Work out the finished part from the listing and answer in its coordinate system (mm). A direction names the side the tool comes from. Give positions to 0.01 mm unless a question says otherwise; leave off trailing zeros. Write each question's results on one line, items separated by ' | '.
from build123d import *

# Parameters (mm, degrees)
EXTRUDE_1_DEPTH     = 5
SKETCH_2_R          = 1.5
CUT_EXTRUDE_1_DEPTH = 202.618451537


with BuildPart() as part:
    # 草圖1 → 填料-伸長1 (new body)
    with BuildSketch(Plane(origin=(0, 0, 0), x_dir=(1, 0, 0), z_dir=(0, 1, 0))):
        Polygon((173, -65), (185, -65), (185, -35), (173, -35), (173, 35), (185, 35), (185, 65), (173, 65), (173, 80), (-173, 80), (-173, 65), (-185, 65), (-185, 35), (-173, 35), (-173, -35), (-185, -35), (-185, -65), (-173, -65), (-173, -80), (173, -80), align=None)
    extrude(amount=EXTRUDE_1_DEPTH)

    # 草圖2 → 除料-伸長1 (cut, through all)
    with BuildSketch(Plane(origin=(0, 5, 0), x_dir=(1, 0, 0), z_dir=(0, 1, 0))):
        with Locations(Location((-53.75, 16.75, 0), (0, 0, 270))):
            Circle(SKETCH_2_R)
        with Locations(Location((53.75, 16.75, 0), (0, 0, 90))):
            Circle(SKETCH_2_R)
        with Locations(Location((53.75, -68.5, 0), (0, 0, 270))):
            Circle(SKETCH_2_R)
        with Locations(Location((-53.75, -68.5, 0), (0, 0, 90))):
            Circle(SKETCH_2_R)
        with BuildLine():
            Line((-173, -20), (-163, -20))
            ThreePointArc((-163, -20), (-155.928932188, -17.071067812), (-153, -10))
            Line((-153, -10), (-153, 10))
            ThreePointArc((-153, 10), (-155.928932188, 17.071067812), (-163, 20))
            Line((-163, 20), (-173, 20))
            Line((-173, 20), (-173, -20))
        make_face()
        with BuildLine():
            Line((173, 20), (163, 20))
            ThreePointArc((163, 20), (155.928932188, 17.071067812), (153, 10))
            Line((153, 10), (153, -10))
            ThreePointArc((153, -10), (155.928932188, -17.071067812), (163, -20))
            Line((163, -20), (173, -20))
            Line((173, -20), (173, 20))
        make_face()
    extrude(amount=-CUT_EXTRUDE_1_DEPTH, mode=Mode.SUBTRACT)


solid = part.part
1. Straight lines are drawn through the part: line 1 (X direction, y = 1.3, z = 68.5); line 2 (X direction, y = 0.85, z = 2.5); line 3 (X direction, y = 3.8, z = 22). For each, find the intervals that lie inside material, in ascending order. Write a range as [from, to].
Answer list:
line 1: [-173, -55.25], [-52.25, 52.25], [55.25, 173] | line 2: [-153, 153] | line 3: [-173, 173]
2. A cutting plane is placed at A-A, the plane y = 3.1. State how many separate pieces and enclosed holes the cut face has, then the cut area to 3 significant figures.
Answer list:
separate pieces: 1 | enclosed holes: 4 | area: 55,300 mm^2
3. A tool of negligible diameter and unlimited length cuts with its end or side. For faces 1 (the face through (156.01, 2.54, -17.15)), 2 (the face through (-156.01, 2.54, 17.15)), 3 (the face through (-3, 0, -1)), from which of +Z, -Z, +X, -X, +Y, -Y can it reach the whole face along a straight path? Write none if from no direction.
Answer list:
face 1: +X, +Y, -Y | face 2: -X, +Y, -Y | face 3: +Z, -Z, +X, -X, -Y
4. Given P1, Ø2.5, axis at x = -178.5, y = 2, coming from the -Z side; P2, Ø2, axis at y = 4, z = 22, coming from the +X side; P3, Ø4, axis at x = 53.75, z = 68.5, coming from the +Y side; P4, Ø1.5, axis at y = 2.5, z = -71, coming from the -X side, each flat-ended and moving along its own axis, determine where each tip first touches the part or whether it passes through.
Answer list:
P1: z = -65 | P2: x = 173 | P3: y = 5 | P4: x = -173
5. Determine the mould class of faces 4 (the face through (155.85, 2.54, 16.99)), 5 (the face through (-3, 5, -1)) for opening direction Z: +Z half, -Z half, draft (parallel to the pull), parting line (faces both ways), or undercut.
Answer list:
face 4: undercut | face 5: draft
